Here's how the part is built. I have some questions about the finished solid (model axes, mm). Face numbers are marked on the shaded views. A direction names the side the tool comes from. Round coordinates to 2 decimals unless told otherwise and drop trailing zeros. Loops run counter-clockwise (first coordinate to the right, second up) from the corner with the lowest first, then second, coordinate; pieces in that order, holes last. Notation, with made-up numbers: (11, -25.75) -> (15, -25.75) arc R18 ccw to (15, 5.25) -> close; hole circle Ø1 at (46.5, 28). An arc over 180 degrees is marked (long way). Use one line per item in the form item = value. Start each with the question number.
Item 1: If we section it at A-A (y = 0): Write out the boundary of the cut face in (x, z), then the cut area to 3 significant figures.
Item 2: If we section it at D-D (y = -18.5): Write out the boundary of the cut face in (x, z).
Item 3: If we section it at C-C (z = 20.25): Write out the boundary of the cut face in (x, y), then the cut area to 3 significant figures.
Item 4: For the marked faces 1, 2 and 3, which set-ups out of +Z, -Z, +X, -X, +Y, -Y let a thin tool reach every point of the face, with its end or its side?
Item 5: I'm going to push flat-ended pins straight in: pin 1 Ø4 at (y, z) = (-5.5, 15) entering from -X; pin 2 Ø2 at (y, z) = (20, 14) entering from +X; pin 3 Ø12 at (y, z) = (-16, 12.5) entering from +X. Where does each tip first touch, or does it pass through?
Item 6: Thinking about a two-plate mould opening in Y: for the marked faces 4, 5 and 6, which applies, released by +Y, released by -Y, zero draft, split by the parting line, or undercut?
Item 7: If I drill on L1, parallel to Y at x = 0, z = 15.25; L2, parallel to Y at x = 0, z = 4.5; L3, parallel to Z at x = 4, y = -9.5, over which ranges is the centre line in solid material (lowest first)? Write a range as [from, to].
```python
from build123d import *

# Parameters (mm, degrees)
F0_R     = 24.95
F1_DEPTH = 6
F2_R     = 30
F3_DEPTH = 10
F4_R     = 24.95
F5_DEPTH = 6
F6_R     = 20
F7_DEPTH = 22.001
F8_R     = 24.95
F8_R_2   = 10
F9_DEPTH = 10


with BuildPart() as f1:
    # F0 (on Top) → F1 (new body)
    with BuildSketch(Plane.XY):
        Circle(F0_R)
    extrude(amount=F1_DEPTH)

    # F2 (on face) → F3 (join)
    with BuildSketch(Plane.XY.offset(6)):
        Circle(F2_R)
    extrude(amount=F3_DEPTH)

    # F4 (on face) → F5 (join)
    with BuildSketch(Plane.XY.offset(16)):
        Circle(F4_R)
    extrude(amount=F5_DEPTH)

    # F6 (on face) → F7 (cut, through all)
    with BuildSketch(Plane.XY.offset(22)):
        Circle(F6_R)
    extrude(amount=-F7_DEPTH, mode=Mode.SUBTRACT)

    # F8 (on face) → F9 (join)
    with BuildSketch(Plane(origin=(0, 0, 0), x_dir=(1, 0, 0), z_dir=(0, 0, -1))):
        Circle(F8_R)
        Circle(F8_R_2, mode=Mode.SUBTRACT)
    extrude(amount=-F9_DEPTH)


solid = f1.part
```
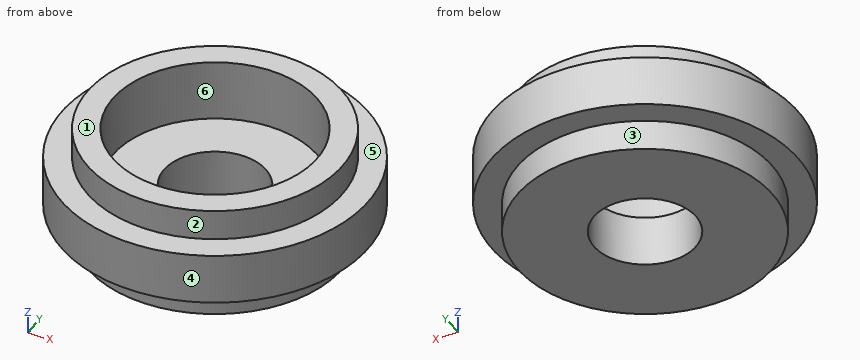
Values found:
q1.outline = (-30, 6) -> (-24.95, 6) -> (-24.95, 0) -> (-10, 0) -> (-10, 10) -> (-20, 10) -> (-20, 22) -> (-24.95, 22) -> (-24.95, 16) -> (-30, 16) -> close; (10, 0) -> (24.95, 0) -> (24.95, 6) -> (30, 6) -> (30, 16) -> (24.95, 16) -> (24.95, 22) -> (20, 22) -> (20, 10) -> (10, 10) -> close
q1.area = 519 mm2
q2.outline = (-23.62, 6) -> (-16.74, 6) -> (-16.74, 0) -> (16.74, 0) -> (16.74, 6) -> (23.62, 6) -> (23.62, 16) -> (16.74, 16) -> (16.74, 22) -> (7.6, 22) -> (7.6, 10) -> (-7.6, 10) -> (-7.6, 22) -> (-16.74, 22) -> (-16.74, 16) -> (-23.62, 16) -> close
q3.outline = circle Ø49.9 at (0, 0); hole circle Ø40 at (0, 0)
q3.area = 699 mm2
q4.face_1 = +Z, +X, -X, +Y, -Y
q4.face_2 = +Z
q4.face_3 = -Z
q5.pin_1 = -29.8
q5.pin_2 = 23.22
q5.pin_3 = 28.28
q6.face_4 = split by the parting line
q6.face_5 = zero draft
q6.face_6 = undercut
q7.L1 = [-30, -20], [20, 30]
q7.L2 = [-24.95, -10], [10, 24.95]
q7.L3 = [0, 10]
